Input: part model. Units: mm. Frame: model coordinates. A direction names the side the tool comes from. Coordinates: 2 decimals unless noted, no trailing zeros. Write each loop counter-clockwise with the first axis right and the second up, starting at its lowest first coordinate (ties: lowest second). Pieces come first, ordered by that corner, then holes.
1) Section query C-C (z = 2.25). Output: boundary loops of the cut face in (x, y).
2) Section query B-B (y = -8.25). Output: boundary loops of the cut face in (x, z).
3) Set-up query: faces 1 (the flat face through (5.08, 0, 3)), 2 (the flat face through (0, 10.08, 3)). Return all of +Z, -Z, +X, -X, +Y, -Y with unobstructed straight access to the full face (end or side cutting, diameter ignored); none if empty.
4) Section query A-A (x = 5.5). Output: boundary loops of the cut face in (y, z), then the cut area to 3 significant figures.
5) Draft query along Z for faces 3 (the flat face through (0, 0, 6.36)), 4 (the flat face through (-8.56, -8.6, 3.14)), 5 (the flat face through (8, 9.58, 3)), 6 (the flat face through (0, 0, 0)). Return one class per face: pulls with the +Z half, pulls with the -Z half, needs draft (parallel to the pull), parting line crosses it, or undercut.
6) Pin query (flat end, axial travel): pin 1 Ø2.5 at (y, z) = (4.5, 3) entering from +X. Return the tip coordinate at first contact, or that it passes through.
7) Section query D-D (y = 0). Output: boundary loops of the cut face in (x, z).
8) Line query: L1, parallel to Y at x = 7.25, z = 2.75; L2, parallel to Z at x = 7.5, y = -5.5; L3, parallel to X at y = 3, z = 5.75. Output: solid intervals per line, ascending.
from build123d import *

# Parameters (mm, degrees)
SKETCH_1_W          = 20.16
SKETCH_1_H          = 20.16
EXTRUDE_1_DEPTH     = 6.36
SKETCH_2_W          = 5.36
SKETCH_2_H          = 19.16
CUT_EXTRUDE_1_DEPTH = 5
CHAMFER_1_SIZE      = 3


with BuildPart() as part:
    # 草图1 → 凸台-拉伸1 (new body)
    with BuildSketch(Plane.XY):
        Rectangle(SKETCH_1_W, SKETCH_1_H)
    extrude(amount=EXTRUDE_1_DEPTH)

    # 草图2 → 切除-拉伸1 (cut)
    with BuildSketch(Plane(origin=(10.08, 0, 0), x_dir=(0, 0, -1), z_dir=(1, 0, 0))):
        with Locations((-3.18, 0)):
            Rectangle(SKETCH_2_W, SKETCH_2_H)
    extrude(amount=-CUT_EXTRUDE_1_DEPTH, mode=Mode.SUBTRACT)

    # 倒角1
    chamfer_1_edges = [part.edges().sort_by_distance(p)[0] for p in [
        (-10.08, -10.08, 3.18),
    ]]
    chamfer(chamfer_1_edges, length=CHAMFER_1_SIZE)


solid = part.part
Answer:
1. outline: (-10.08, -7.08) - (-7.08, -10.08) - (10.08, -10.08) - (10.08, -9.58) - (5.08, -9.58) - (5.08, 9.58) - (10.08, 9.58) - (10.08, 10.08) - (-10.08, 10.08) - close
2. outline: (-8.91, 0) - (10.08, 0) - (10.08, 0.5) - (5.08, 0.5) - (5.08, 5.86) - (10.08, 5.86) - (10.08, 6.36) - (-8.91, 6.36) - close
3. face 1: +X
3. face 2: +Z, -Z, +X, -X, +Y
4. outline: (-10.08, 0) - (10.08, 0) - (10.08, 6.36) - (-10.08, 6.36) - close; hole (-9.58, 0.5) - (9.58, 0.5) - (9.58, 5.86) - (-9.58, 5.86) - close
4. area: 25.5 mm2
5. face 3: pulls with the +Z half
5. face 4: needs draft
5. face 5: undercut
5. face 6: pulls with the -Z half
6. pin 1: stops at x = 5.08
7. outline: (-10.08, 0) - (10.08, 0) - (10.08, 0.5) - (5.08, 0.5) - (5.08, 5.86) - (10.08, 5.86) - (10.08, 6.36) - (-10.08, 6.36) - close
8. L1: y = -10.08 to -9.58, 9.58 to 10.08
8. L2: z = 0 to 0.5, 5.86 to 6.36
8. L3: x = -10.08 to 5.08
